Input: part model. Units: mm. Frame: model coordinates. A direction names the side the tool comes from. Coordinates: 2 decimals unless noted, no trailing zeros. Write each loop counter-clockwise with the first axis right and the second up, starting at its lowest first coordinate (ties: lowest second). Pieces come first, ordered by that corner, then holes. Notation, with made-up numbers: M 26.25,52 L 50.25,52 A31 cw 50.25,89 Z; hole C 41,-0.5 d7. An arc over 180 degrees is marked long. Use CSV: the item, a comma, the result in double quotes.
```python
from build123d import *

# Parameters (mm, degrees)
F0_W            = 210
F0_H            = 225
F1_DEPTH        = 25
F3_DEPTH        = 95
F4_R            = 37.5
F5_DEPTH        = 10
F5_DEPTH_BACK   = 127
F6_R            = 37.5
F7_DEPTH        = 10
F7_DEPTH_BACK   = 127
F8_W            = 60
F8_H            = 60
F9_DEPTH        = 10
F10_R           = 10
F12_DEPTH       = 20
F14_D           = 15
F14_CBORE_D     = 30
F14_CBORE_DEPTH = 10
F15_R           = 10
F16_R           = 19.5
F17_DEPTH       = 235.001
F18_R           = 24.199633
F19_DEPTH       = 220.001
F20_SIZE        = 2
F21_R           = 10


with BuildPart() as f1:
    # F0 (on Top) → F1 (new body)
    with BuildSketch(Plane.XY):
        Rectangle(F0_W, F0_H)
    extrude(amount=F1_DEPTH)

    # F2 (on face) → F3 (join)
    with BuildSketch(Plane.XY.offset(25)):
        with BuildLine():
            Line((-71, -32.5), (-71, -112.5))
            Line((-71, -112.5), (-56, -112.5))
            Line((-56, -112.5), (-56, -46.481817))
            ThreePointArc((-56, -46.481817), (7.488853, -14.988853), (38.981817, 48.5))
            Line((38.981817, 48.5), (105, 48.5))
            Line((105, 48.5), (105, 63.5))
            Line((105, 63.5), (25, 63.5))
            ThreePointArc((25, 63.5), (-3.117749, -4.382251), (-71, -32.5))
        make_face()
    extrude(amount=F3_DEPTH)

    # F4 (on face) → F5 (join, two sides)
    with BuildSketch(Plane.XZ.offset(112.5)) as f5_sk:
        with Locations((-63.5, 120)):
            Circle(F4_R)
    extrude(amount=F5_DEPTH)
    extrude(f5_sk.sketch, amount=-F5_DEPTH_BACK)

    # F6 (on face) → F7 (join, two sides)
    with BuildSketch(Plane.YZ.offset(105)) as f7_sk:
        with Locations((56, 120)):
            Circle(F6_R)
    extrude(amount=F7_DEPTH)
    extrude(f7_sk.sketch, amount=-F7_DEPTH_BACK)

    # F8 (on face) → F9 (join)
    with BuildSketch(Plane.XY.offset(25)):
        with Locations((75, -82.5)):
            Rectangle(F8_W, F8_H)
    extrude(amount=F9_DEPTH)

    # F10
    f10_edges = [f1.edges().sort_by_distance(p)[0] for p in [
        (45, -52.5, 30),
    ]]
    fillet(f10_edges, radius=F10_R)

    # F11 (on face) → F12 (cut)
    with BuildSketch(Plane.XY.offset(25)):
        with BuildLine():
            ThreePointArc((46.575508, 39.5), (13.852814, -21.352814), (-47, -54.075508))
            Line((-47, -54.075508), (-47, -103.5))
            Line((-47, -103.5), (36, -103.5))
            Line((36, -103.5), (36, -62.5))
            ThreePointArc((36, -62.5), (41.564971, -49.064971), (55, -43.5))
            Line((55, -43.5), (96, -43.5))
            Line((96, -43.5), (96, 39.5))
            Line((96, 39.5), (46.575508, 39.5))
        make_face()
    extrude(amount=-F12_DEPTH, mode=Mode.SUBTRACT)

    # F14 (through all)
    with Locations(Plane.XY.offset(35)):
        with Locations((75, -82.5)):
            CounterBoreHole(F14_D / 2, F14_CBORE_D / 2, F14_CBORE_DEPTH)

    # F15
    f15_edges = [f1.edges().sort_by_distance(p)[0] for p in [
        (46.575508, 39.5, 15),
        (-47, -54.075508, 15),
        (-47, -103.5, 15),
        (96, 39.5, 15),
        (96, -43.5, 15),
        (36, -103.5, 15),
    ]]
    fillet(f15_edges, radius=F15_R)

    # F16 (on face) → F17 (cut, through all)
    with BuildSketch(Plane.XZ.offset(122.5)):
        with Locations((-63.5, 120)):
            Circle(F16_R)
    extrude(amount=-F17_DEPTH, mode=Mode.SUBTRACT)

    # F18 (on face) → F19 (cut, through all)
    with BuildSketch(Plane.YZ.offset(115)):
        with Locations((56, 120)):
            Circle(F18_R)
    extrude(amount=-F19_DEPTH, mode=Mode.SUBTRACT)

    # F20
    f20_edges = [f1.edges().sort_by_distance(p)[0] for p in [
        (-83, -122.5, 120),
        (115, 31.800367, 120),
        (-22, 31.800367, 120),
        (-83, 14.5, 120),
    ]]
    chamfer(f20_edges, length=F20_SIZE)

    # F21
    f21_edges = [f1.edges().sort_by_distance(p)[0] for p in [
        (-105, -112.5, 12.5),
        (105, -112.5, 17.5),
        (105, 112.5, 12.5),
        (-105, 112.5, 12.5),
    ]]
    fillet(f21_edges, radius=F21_R)


solid = f1.part
```
1. Access query for faces 5 (the flat face through (45, -88, 30)), 6 (the flat face through (68, -69, 35)), 7 (the flat face through (-47, 14.5, 104)), 8 (the flat face through (96, -2, 15)). Directions: +Z, -Z, +X, -X, +Y, -Y. A direction counts if a zero-diameter tool reaches every point of the face in a straight line with its end or side. Return the directions, or none.
Resolved:
face 5,"+Z, -Y"
face 6,"+Z, +X, -Y"
face 7,"+Z, -X, +Y"
face 8,"none"
2. Material intervals for line 1 (Z direction, x = -63.5, y = -18); line 2 (Z direction, x = 71, y = 56); line 3 (Y direction, x = 66, z = 18), sorted ascending. Write a range as [from, to].
Resolved:
line 1,"z = [0, 25], [82.5, 100.5], [139.5, 157.5]"
line 2,"z = [0, 95.8], [144.2, 157.5]"
line 3,"y = [-112.5, -43.5], [39.5, 112.5]"
3. Mould query, pull axis X, two halves, no side actions, for faces 1 (the flat face through (-105, -1, 12)), 2 (the flat face through (72, 48.5, 54)), 3 (the cylindrical face through (-77.87, -54.93, 133.18)), 4 (the flat face through (42, -50, 25)). Classes: pulls with the +X half, pulls with the -X half, needs draft (parallel to the pull), parting line crosses it, or undercut.
Resolved:
face 1,"pulls with the -X half"
face 2,"needs draft"
face 3,"undercut"
face 4,"undercut"
4. Section C-C (x = -63.5). Return loops of the section in (y, z), then the cut area to 3 significant figures.
Resolved:
outline,"M -122.5,82.5 L -112.5,82.5 L -112.5,0 L 112.5,0 L 112.5,25 L -32.21,25 L -32.21,82.5 L 14.5,82.5 L 14.5,98.5 L 12.5,100.5 L -120.5,100.5 L -122.5,98.5 Z; M -122.5,141.5 L -120.5,139.5 L 12.5,139.5 L 14.5,141.5 L 14.5,157.5 L -122.5,157.5 Z"
area,"15,200 mm^2"
5. Section D-D (z = 49). Return loops of the section in (x, y), then the cut area to 3 significant figures.
Resolved:
outline,"M -71,-112.5 L -56,-112.5 L -56,-46.48 A111 ccw 38.98,48.5 L 105,48.5 L 105,63.5 L 25,63.5 A96 cw -71,-32.5 Z"
area,"4,400 mm^2"
6. Section B-B (x = 75). Return loops of the section in (y, z).
Resolved:
outline,"M -112.5,0 L -90,0 L -90,25 L -97.5,25 L -97.5,35 L -112.5,35 Z; M -75,0 L 112.5,0 L 112.5,25 L 63.5,25 L 63.5,83.26 A37.5 ccw long 48.5,83.26 L 48.5,25 L 39.5,25 L 39.5,5 L -43.5,5 L -43.5,25 L -52.5,25 L -52.5,35 L -67.5,35 L -67.5,25 L -75,25 Z; hole C 56,120 d48.4"
7. Contact query for flat-ended pins moving along their axis: pin 1 Ø22.5 at (y, z) = (41.5, 122.5) entering from -X; pin 2 Ø6 at (x, z) = (91, 61) entering from -Y; pin 3 Ø2 at (y, z) = (-83, 52) entering from +X. Output: stop coordinate, or through.
Resolved:
pin 1,"stops at x = -21.76"
pin 2,"stops at y = 48.5"
pin 3,"stops at x = -56"
8. Section A-A (y = -82.5). Return loops of the section in (x, z).
Resolved:
outline,"M -105,0 L 67.5,0 L 67.5,25 L 60,25 L 60,35 L 45,35 L 45,25 L 36,25 L 36,5 L -47,5 L -47,25 L -56,25 L -56,83.26 A37.5 ccw long -71,83.26 L -71,25 L -105,25 Z; M 82.5,0 L 105,0 L 105,35 L 90,35 L 90,25 L 82.5,25 Z; hole C -63.5,120 d39"
